Can you work these out from the model? Positions are in its coordinate system, mm. A direction names the side the tool comes from. Round coordinates to 2 decimals unless told otherwise and drop trailing zeros. Loops run counter-clockwise (first coordinate to the right, second up) from the corner with the lowest first, then second, coordinate; pieces in that order, holes last.
(1) Thinking about a two-plate mould opening in X: for faces 1 (the face through (125, -83, 102.5)), 2 (the face through (-101.91, 585.59, 593.84)), 3 (the face through (27.5, -81, 52)), which applies, released by +X, released by -X, zero draft, split by the parting line, or undercut?
(2) I want a section at A-A on z = 84.5. Write out the boundary of the cut face in (x, y).
(3) Will these pins go through, and if not, where does the flat tip stop? pin 1 Ø12 at (x, z) = (-7, 211.5) entering from +Y; pin 2 Ø24 at (x, z) = (74.5, 27.5) entering from +Y; pin 3 Ø7.5 at (x, y) = (72.5, -139.5) entering from -Z; pin 4 Ø1 at (x, z) = (44, 274) entering from -Y.
(4) If I drill on line 1 along Y through (x, z) = (-100, 597.5); line 2 along Z through (x, y) = (-119, 673); line 3 along Y through (x, z) = (58.5, 219), over which ranges is the centre line in solid material (lowest first)?
(5) I want a section at B-B on y = 325.5. Write out the boundary of the cut face in (x, z).
(6) Which directions (+Z, -Z, +X, -X, +Y, -Y) give clear straight access to the entire face, cutting with the end or side of a thin tool? Please do faces 4 (the face through (30, -81, 51)), 5 (the face through (101.35, 283.56, 612.77)), 6 (the face through (15, -79, 102.5)).
(7) I want a section at C-C on x = -117. Write out the boundary of the cut face in (y, z), plus the area to 3 significant figures.
from build123d import *
from build123d.topology import SkipClean

# Parameters (mm, degrees)
CROQUIS1_W              = 140
CROQUIS1_H              = 161
CROQUIS1_W_2            = 80
CROQUIS1_H_2            = 101
SALIENTE_EXTRUIR1_DEPTH = 2.5
CROQUIS2_W              = 85
CROQUIS2_H              = 106
CROQUIS2_W_2            = 80
CROQUIS2_H_2            = 101
SALIENTE_EXTRUIR2_DEPTH = 100
CROQUIS3_R              = 67.935631299
SALIENTE_EXTRUIR3_DEPTH = 100
CROQUIS4_R              = 67.935631299


with BuildPart() as part:
    # Croquis1 → Saliente-Extruir1 (new body)
    with BuildSketch(Plane.XY):
        with Locations((70, -80.5)):
            Rectangle(CROQUIS1_W, CROQUIS1_H)
        with Locations((70, -80.5)):
            Rectangle(CROQUIS1_W_2, CROQUIS1_H_2, mode=Mode.SUBTRACT)
    extrude(amount=SALIENTE_EXTRUIR1_DEPTH)

    # Croquis2 → Saliente-Extruir2 (add)
    with BuildSketch(Plane.XY.offset(2.5)):
        with Locations((70, -80.5)):
            Rectangle(CROQUIS2_W, CROQUIS2_H)
        with Locations((70, -80.5)):
            Rectangle(CROQUIS2_W_2, CROQUIS2_H_2, mode=Mode.SUBTRACT)
    extrude(amount=SALIENTE_EXTRUIR2_DEPTH)

    # Croquis3 → Saliente-Extruir3 (add)
    with BuildSketch(Plane.XY.offset(102.5)):
        with Locations(Location((70, -80.5, 0), (0, 0, 128.725665443))):
            Circle(CROQUIS3_R)
    extrude(amount=SALIENTE_EXTRUIR3_DEPTH)

    # Barrer1: sweep along a curve in space
    with SkipClean():  # the faces are left unmerged after this step: merging them gives an invalid solid
        with BuildLine() as barrer1_path:
            Line((70, -80.5, 202.5), (70, -80.5, 482.5))
            ThreePointArc((70, -80.5, 482.5), (70, -59.997474683, 531.997474683), (70, -10.5, 552.5))
            Line((70, -10.5, 552.5), (70, 569.5, 552.5))
            ThreePointArc((70, 569.5, 552.5), (49.497474683, 618.997474683, 552.5), (0, 639.5, 552.5))
            Line((0, 639.5, 552.5), (-201.005050634, 639.5, 552.5))
            ThreePointArc((-201.005050634, 639.5, 552.5), (-227.792890899, 639.5, 557.828432724), (-250.502525317, 639.5, 573.002525317))
            Line((-360, 639.5, 682.5), (-250.502525317, 639.5, 573.002525317))
        # Croquis4 → Barrer1 (sweep)
        with BuildSketch(Plane.XY.offset(202.5)):
            with Locations((70, -80.5)):
                Circle(CROQUIS4_R)
        sweep(path=barrer1_path.line)


solid = part.part
Filled sheet:
1. face 1: zero draft
1. face 2: undercut
1. face 3: released by -X
2. outline: (27.5, -133.5) - (112.5, -133.5) - (112.5, -27.5) - (27.5, -27.5) - close; hole (30, -131) - (110, -131) - (110, -30) - (30, -30) - close
3. pin 1: passes through
3. pin 2: stops at y = -27.5
3. pin 3: stops at z = 0
3. pin 4: stops at y = -143.47
4. line 1: y = 588.61 to 690.39
4. line 2: z = 493.4 to 611.6
4. line 3: y = -147.46 to -13.54
5. outline: circle Ø135.87 at (70, 552.5)
6. face 4: -Z
6. face 5: none
6. face 6: -X, +Y, -Y
7. outline: circle Ø135.87 at (639.5, 552.5)
7. area: 14,500 mm2
